The model under review builds one solid part; all positions refer to its coordinate system, in mm. Round coordinates to 2 decimals unless told otherwise and drop trailing zeros. Order: outer loops, then holes, each group sorted by start corner. A loop starts at its lowest first (then second) coordinate and runs counter-clockwise, first axis right, second up. Notation, with made-up numbers: M -37,-24 L -14,-24 A31 ccw -14,5 Z; hole C -19.75,-10.5 d8. An arc over 180 degrees is marked long. Answer as a JSON object with one key per item and string values. Group by question number.
1) The part is to be moulded in two halves that separate along X. For faces 1 (the cylindrical face through (-1.86, 54.87, -0.04)), 2 (the cylindrical face through (64.86, 78.51, -0.04)), 3 (the flat face through (-1, 23, 3.175)), 4 (the cylindrical face through (30.99, 31.42, -0.04)), say which applies: +X half, -X half, draft (parallel to the pull), parting line (faces both ways), or undercut.
2) Consider section C-C, the plane y = 47. Write out the cut boundary in (x, z) (3 decimals), then the cut area to 3 significant figures.
3) Consider section D-D, the plane z = 1.75. Count the separate pieces of the cut face and the enclosed holes in it, then the cut area to 3 significant figures.
4) Consider section A-A, the plane y = 0. Write out the cut boundary in (x, z) (1 decimal).
5) Insertion check: pin 1 Ø3 at (x, y) = (-38.66, -18.31) entering from +Z. The pin has a flat end and moves straight along its axis. Give the tip position at first contact, or say it passes through.
6) To check wall thickness, follow line 1 (Y direction, x = 0, z = -1.25); line 2 (X direction, y = -18, z = 1.75) (3 decimals); line 3 (X direction, y = 35.5, z = -0.5) (3 decimals). State the ranges of each line that lie inside material, in increasing order.
7) Consider section B-B, the plane x = 0. Write out the cut boundary in (y, z) (1 decimal), then the cut area to 3 significant figures.
```python
from build123d import *

# Parameters (mm, degrees)
SKETCH1_W           = 133.35
SKETCH1_H           = 117.475
SKETCH1_R           = 14.2748
SKETCH1_R_2         = 9.525
SKETCH1_R_3         = 14.2875
SKETCH1_R_4         = 4.064
SKETCH1_R_5         = 2.667
BOSS_EXTRUDE1_DEPTH = 3.175
FILLET1_R           = 6.35


with BuildPart() as part:
    # Sketch1 → Boss-Extrude1 (new, symmetric)
    with BuildSketch(Plane.XY):
        with Locations((0, 21.6789)):
            Rectangle(SKETCH1_W, SKETCH1_H)
        with Locations((0, 40.7162)):
            Circle(SKETCH1_R, mode=Mode.SUBTRACT)
        with Locations((33.0581, 40.7162)):
            Circle(SKETCH1_R_2, mode=Mode.SUBTRACT)
        with Locations((-33.0581, 40.7162)):
            Circle(SKETCH1_R_2, mode=Mode.SUBTRACT)
        Circle(SKETCH1_R_3, mode=Mode.SUBTRACT)
        with Locations((-57.15, 70.8914)):
            Circle(SKETCH1_R_4, mode=Mode.SUBTRACT)
        with Locations((-55.626, -30.2006)):
            Circle(SKETCH1_R_4, mode=Mode.SUBTRACT)
        with Locations((57.15, 70.8914)):
            Circle(SKETCH1_R_4, mode=Mode.SUBTRACT)
        with Locations((55.626, -30.2006)):
            Circle(SKETCH1_R_4, mode=Mode.SUBTRACT)
        with Locations((38.6588, -18.3134)):
            Circle(SKETCH1_R_5, mode=Mode.SUBTRACT)
        with Locations((-38.6588, -18.3134)):
            Circle(SKETCH1_R_5, mode=Mode.SUBTRACT)
        with Locations((-31.75, 70.5866)):
            Circle(SKETCH1_R_5, mode=Mode.SUBTRACT)
        with Locations((31.75, 70.5866)):
            Circle(SKETCH1_R_5, mode=Mode.SUBTRACT)
    extrude(amount=BOSS_EXTRUDE1_DEPTH, both=True)

    # Fillet1
    fillet1_edges = [part.edges().sort_by_distance(p)[0] for p in [
        (66.675, -37.0586, 0),
        (-66.675, -37.0586, 0),
        (-66.675, 80.4164, 0),
        (66.675, 80.4164, 0),
    ]]
    fillet(fillet1_edges, radius=FILLET1_R)


solid = part.part
```
Results list:
{
 "1": {"face 1": "undercut", "face 2": "+X half", "face 3": "draft", "face 4": "undercut"},
 "2": {"outline": "M -66.675,-3.175 L -40.216,-3.175 L -40.216,3.175 L -66.675,3.175 Z; M -25.9,-3.175 L -12.817,-3.175 L -12.817,3.175 L -25.9,3.175 Z; M 12.817,-3.175 L 25.9,-3.175 L 25.9,3.175 L 12.817,3.175 Z; M 40.216,-3.175 L 66.675,-3.175 L 66.675,3.175 L 40.216,3.175 Z", "area": "502 mm^2"},
 "3": {"separate pieces": "1", "enclosed holes": "12", "area": "13,500 mm^2"},
 "4": {"outline": "M -66.7,-3.2 L -14.3,-3.2 L -14.3,3.2 L -66.7,3.2 Z; M 14.3,-3.2 L 66.7,-3.2 L 66.7,3.2 L 14.3,3.2 Z"},
 "5": {"pin 1": "through"},
 "6": {"line 1": "-37.06 to -14.29, 14.29 to 26.44, 54.99 to 80.42", "line 2": "-66.675 to -41.307, -36.01 to 36.01, 41.307 to 66.675", "line 3": "-66.675 to -41.028, -25.088 to -13.288, 13.288 to 25.088, 41.028 to 66.675"},
 "7": {"outline": "M -37.1,-3.2 L -14.3,-3.2 L -14.3,3.2 L -37.1,3.2 Z; M 14.3,-3.2 L 26.4,-3.2 L 26.4,3.2 L 14.3,3.2 Z; M 55,-3.2 L 80.4,-3.2 L 80.4,3.2 L 55,3.2 Z", "area": "383 mm^2"}
}
